from build123d import *

# Parameters (mm, degrees)
SKETCH3_W           = 25
SKETCH3_H           = 12
BOSS_EXTRUDE1_DEPTH = 4
SINGLE_HORN_DEPTH   = 2.5
SKETCH4_W           = 4
SKETCH4_H           = 12
BOSS_EXTRUDE2_DEPTH = 43.5
SKETCH5_W           = 25
SKETCH5_H           = 12
BOSS_EXTRUDE4_DEPTH = 4
SKETCH6_R           = 2.75
CUT_EXTRUDE3_DEPTH  = 4
FILLET1_R           = 5
DOUBLE_HORN_DEPTH   = 2.5


with BuildPart() as part:
    # Sketch3 → Boss-Extrude1 (new body)
    with BuildSketch(Plane(origin=(0, 0, 0), x_dir=(1, 0, 0), z_dir=(0, 1, 0))):
        with Locations((5.890813757, 0)):
            Rectangle(SKETCH3_W, SKETCH3_H)
    extrude(amount=-BOSS_EXTRUDE1_DEPTH)

    # Sketch1 → single horn (cut)
    with BuildSketch(Plane(origin=(0, 0, 0), x_dir=(1, 0, 0), z_dir=(0, 1, 0))):
        with BuildLine():
            Line((14.254126854, 1.962408156), (2.029090374, 3.299759756))
            ThreePointArc((2.029090374, 3.299759756), (-3.8737091, 0), (2.029090374, -3.299759756))
            Line((2.029090374, -3.299759756), (14.254126854, -1.962408156))
            ThreePointArc((14.254126854, -1.962408156), (16.21653501, 0), (14.254126854, 1.962408156))
        make_face()
    extrude(amount=-SINGLE_HORN_DEPTH, mode=Mode.SUBTRACT)

    # Sketch4 → Boss-Extrude2 (add)
    with BuildSketch(Plane.XZ.offset(4)):
        with Locations((20.390813757, 0)):
            Rectangle(SKETCH4_W, SKETCH4_H)
    extrude(amount=-BOSS_EXTRUDE2_DEPTH)

    # Sketch5 → Boss-Extrude4 (add)
    with BuildSketch(Plane(origin=(0, 39.5, 0), x_dir=(1, 0, 0), z_dir=(0, 1, 0))):
        with Locations((5.890813757, 0)):
            Rectangle(SKETCH5_W, SKETCH5_H)
    extrude(amount=-BOSS_EXTRUDE4_DEPTH)

    # Sketch6 → Cut-Extrude3 (cut)
    with BuildSketch(Plane(origin=(0, 39.5, 0), x_dir=(1, 0, 0), z_dir=(0, 1, 0))):
        Circle(SKETCH6_R)
    extrude(amount=-CUT_EXTRUDE3_DEPTH, mode=Mode.SUBTRACT)

    # Fillet1
    fillet1_edges = [part.edges().sort_by_distance(p)[0] for p in [
        (-6.609186243, 37.5, 6),
        (-6.609186243, 37.5, -6),
        (-6.609186243, -2, -6),
        (-6.609186243, -2, 6),
    ]]
    fillet(fillet1_edges, radius=FILLET1_R)

    # Sketch11 → double horn (cut)
    with BuildSketch(Plane(origin=(22.390813757, 0, 0), x_dir=(0, 0, -1), z_dir=(1, 0, 0))):
        with BuildLine():
            Line((-2.154521604, 32.171561508), (-3.615323039, 20.099129755))
            ThreePointArc((-3.615323039, 20.099129755), (-4.309876098, 17.868064822), (-3.738508691, 15.602321242))
            Line((-3.738508691, 15.602321242), (-2.154521604, 3.109591283))
            ThreePointArc((-2.154521604, 3.109591283), (0.000957171, 0.954112508), (2.156435946, 3.109591283))
            Line((2.156435946, 3.109591283), (3.615323039, 15.400870245))
            ThreePointArc((3.615323039, 15.400870245), (4.311420307, 17.775024288), (3.5878108, 20.140938088))
            Line((3.5878108, 20.140938088), (2.156435946, 32.171561508))
            ThreePointArc((2.156435946, 32.171561508), (0.000957171, 34.327040283), (-2.154521604, 32.171561508))
        make_face()
    extrude(amount=-DOUBLE_HORN_DEPTH, mode=Mode.SUBTRACT)


solid = part.part
Design review of the part built by this model. Coordinates are the model's own, in mm. A direction names the side the tool comes from. Give positions to 0.01 mm unless a question says otherwise; leave off trailing zeros. Order: outer loops, then holes, each group sorted by start corner. A loop starts at its lowest first (then second) coordinate and runs counter-clockwise, first axis right, second up.
1. Mouldability with a two-part tool opening along Y and no side actions: class faces 1 (the flat face through (8, -4, 0)), 2 (the cylindrical face through (-0.596, 37.528, 2.685)), 3 (the flat face through (18.391, 18, 0)) as +Y half, -Y half, draft (parallel to the pull), parting line (faces both ways), or undercut.
Solution:
face 1: -Y half
face 2: draft
face 3: undercut
2. Add section C-C, the plane x = 0. State the section outline as (y, z) points.
Solution:
outline: (-4, -6) - (0, -6) - (0, -3.87) - (-2.5, -3.87) - (-2.5, 3.87) - (0, 3.87) - (0, 6) - (-4, 6) - close; (35.5, -6) - (39.5, -6) - (39.5, -2.75) - (35.5, -2.75) - close; (35.5, 2.75) - (39.5, 2.75) - (39.5, 6) - (35.5, 6) - close
3. For pin 1 Ø3.5 at (x, z) = (0, 0) entering from +Y; pin 2 Ø2.5 at (y, z) = (15.5, 2) entering from +X, all flat-tipped, find the tip position at first contact; note any pin that passes through.
Solution:
pin 1: stops at y = -2.5
pin 2: stops at x = 19.89
4. Add section B-B, the plane z = 0. State the section outline as (x, y) points, then the cut area to 3 significant figures.
Solution:
outline: (-6.61, -4) - (22.39, -4) - (22.39, 0.95) - (19.89, 0.95) - (19.89, 34.33) - (22.39, 34.33) - (22.39, 39.5) - (2.75, 39.5) - (2.75, 35.5) - (18.39, 35.5) - (18.39, 0) - (16.22, 0) - (16.22, -2.5) - (-3.87, -2.5) - (-3.87, 0) - (-6.61, 0) - close; (-6.61, 35.5) - (-2.75, 35.5) - (-2.75, 39.5) - (-6.61, 39.5) - close
area: 218 mm2
5. Add section D-D, the plane y = 1.5. State the section outline as (x, z) points.
Solution:
outline: (18.39, -6) - (22.39, -6) - (22.39, -1.43) - (19.89, -1.43) - (19.89, 1.43) - (22.39, 1.43) - (22.39, 6) - (18.39, 6) - close
6. Tool access review of faces 4 (the flat face through (19.891, 18, 0)), 5 (the cylindrical face through (16.216, -1.232, 0.043)), 6 (the flat face through (6, 35.5, 0)): name each direction out of +Z, -Z, +X, -X, +Y, -Y from which nothing blocks a thin tool from reaching the whole face with its end or side.
Solution:
face 4: +X
face 5: none
face 6: +Z, -Z, -X
7. Add section A-A, the plane x = 8. State the section outline as (y, z) points, then the cut area to 3 significant figures.
Solution:
outline: (-4, -6) - (0, -6) - (0, -2.65) - (-2.5, -2.65) - (-2.5, 2.65) - (0, 2.65) - (0, 6) - (-4, 6) - close; (35.5, -6) - (39.5, -6) - (39.5, 6) - (35.5, 6) - close
area: 82.8 mm2
8. To check wall thickness, follow L1, parallel to Z at x = 0, y = -0.8; L2, parallel to Y at x = 2.25, z = 5; L3, parallel to Y at x = 3.75, z = -0.5. State the ranges of each line that lie inside material, in increasing order.
Solution:
L1: z = -6 to -3.87, 3.87 to 6
L2: y = -4 to 0, 35.5 to 39.5
L3: y = -4 to -2.5, 35.5 to 39.5
